Design review of the part built by this model. Coordinates are the model's own, in mm. Face numbers are marked on the shaded views. A direction names the side the tool comes from. Coordinates: 2 decimals unless noted, no trailing zeros. Write each loop counter-clockwise with the first axis right and the second up, starting at its lowest first coordinate (ties: lowest second). Pieces come first, ordered by that corner, then holes. Notation, with made-up numbers: (9, 37.5) - (64, 37.5) arc R32 ccw to (64, 71.5) - close; hole circle Ø8 at (20, 82). An arc over 180 degrees is marked (long way). Use a Markdown table: item, result.
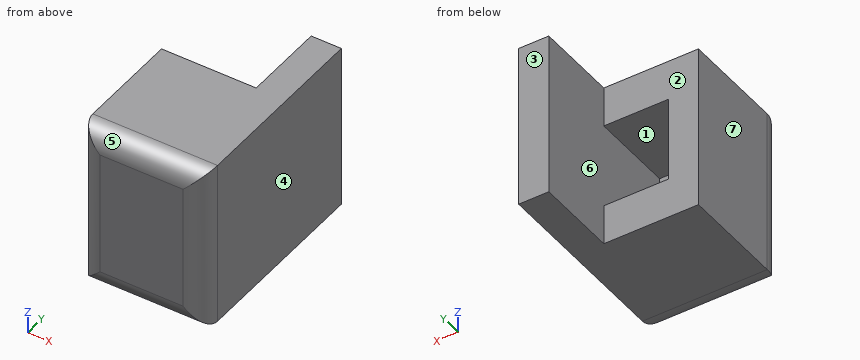
Autodesk Inventor part; units mm, degrees
ref_plane "YZ Plane" through (0, 0, 0) normal (1, 0, 0) x (0, 1, 0)
ref_plane "XZ Plane" through (0, 0, 0) normal (0, 1, 0) x (-1, 0, 0)
ref_plane "XY Plane" through (0, 0, 0) normal (0, 0, 1) x (1, 0, 0)
sketch "Sketch1" plane through (0, 0, 0) normal (0, 1, 0) x (-1, 0, 0)
  line L0 (15, 20) -> (-15, 20)
  line L1 (-15, 20) -> (-15, -20)
  line L2 (-15, -20) -> (15, -20)
  line L3 (15, -20) -> (15, 20)
  line L4 (15, 20) -> (-15, -20) construction
  line L5 (-15, 20) -> (15, -20) construction
  point P0 (0, 0)
  dimension "d0" = 30
  dimension "d1" = 40
extrude "Extrusion1" add sketch "Sketch1" along normal blind 50
sketch "Sketch2" plane through (0, 50, 0) normal (0, 1, 0) x (1, 0, 0)
  line L0 (-7.75, -25.4) -> (7.75, -25.4)
  line L1 (7.75, -25.4) -> (7.75, 25.4)
  line L2 (7.75, 25.4) -> (-7.75, 25.4)
  line L3 (-7.75, 25.4) -> (-7.75, -25.4)
  line L4 (-7.75, -25.4) -> (7.75, 25.4) construction
  line L5 (7.75, -25.4) -> (-7.75, 25.4) construction
  point P0 (0, 0)
  dimension "d4" = 15.5
extrude "Extrusion2" cut sketch "Sketch2" against normal blind 20
sketch "Sketch3" plane through (0, 30, 0) normal (0, 1, 0) x (1, 0, 0)
  line L0 (-7.75, -10.25) -> (7.75, -10.25)
  line L1 (7.75, -10.25) -> (7.75, 10.25)
  line L2 (7.75, 10.25) -> (-7.75, 10.25)
  line L3 (-7.75, 10.25) -> (-7.75, -10.25)
  line L4 (-7.75, -10.25) -> (7.75, 10.25) construction
  line L5 (7.75, -10.25) -> (-7.75, 10.25) construction
  point P0 (0, 0)
  dimension "d7" = 15.5
  dimension "d8" = 20.5
extrude "Extrusion3" cut sketch "Sketch3" against normal blind 20.3
fillet "Fillet1" radius 5 4 edges at (15, 0, 0) (-15, 0, 0) (0, 0, 20) (0, 0, -20)
sketch "Sketch4" plane through (0, 50, 0) normal (0, 1, 0) x (1, 0, 0)
  line L0 (-7.75, -20) -> (-7.75, 20)
  line L1 (-7.75, 20) -> (-15, 20)
  line L2 (-15, 20) -> (-15, -20)
  line L3 (-15, -20) -> (-7.75, -20)
  point P0 (0, 0)
extrude "Extrusion4" cut sketch "Sketch4" against normal blind 20
properties part number "SEGURO DE GUIA DE TAPA PRINCIPAL"
(1) Machinability: for the marked faces 1, 2 and 3, which of the approach directions +Z, -Z, +X, -X, +Y, -Y give a long, thin tool a straight path to every point of the face, cutting with its end or side? Answer none if there is none.
Determined:
| item | result |
|---|---|
| face 1 | +Y |
| face 2 | +Z, -Z, -X, +Y |
| face 3 | +Z, -Z, +X, -X, +Y |
(2) Take a section at A-A on y = 29. Write out the cut boundary in (x, z), and give its area (3 significant figures).
Determined:
| item | result |
|---|---|
| outline | (-15, -20) - (15, -20) - (15, 20) - (-15, 20) - close; hole (-7.75, -10.25) - (7.75, -10.25) - (7.75, 10.25) - (-7.75, 10.25) - close |
| area | 882 mm2 |
(3) For L1, parallel to X at y = 21, z = 5.5; L2, parallel to X at y = 36, z = 6.5; L3, parallel to Y at x = 3.5, z = 6.5, list the stretches that pass through material, from the lowest coordinate up. Write a range as from..to.
Determined:
| item | result |
|---|---|
| L1 | -15..-7.75, 7.75..15 |
| L2 | 7.75..15 |
| L3 | 0..9.7 |
(4) Take a section at B-B on z = -11. Write out the cut boundary in (x, y), and give its area (3 significant figures).
Determined:
| item | result |
|---|---|
| outline | (-15, 5) arc R5 ccw to (-10, 0) - (10, 0) arc R5 ccw to (15, 5) - (15, 50) - (7.75, 50) - (7.75, 30) - (-15, 30) - close |
| area | 1,030 mm2 |
(5) Draft analysis for pull direction X (two halves, no side actions). For the marked faces 4, 5, 6 and 7, state which applies: +X half, -X half, draft (parallel to the pull), parting line (faces both ways), or undercut.
Determined:
| item | result |
|---|---|
| face 4 | +X half |
| face 5 | draft |
| face 6 | undercut |
| face 7 | -X half |
(6) For pin 1 (12.5 mm diameter, centred on x = -3.5, z = 2.5, fed in from +Y); pin 2 (4 mm diameter, centred on x = 2, z = -0.5, fed in from +Y), all flat-tipped, find the tip position at first contact; note any pin that passes through.
Determined:
| item | result |
|---|---|
| pin 1 | y = 30 |
| pin 2 | y = 9.7 |
(7) Take a section at C-C on x = -2.5. Write out the cut boundary in (y, z).
Determined:
| item | result |
|---|---|
| outline | (0, -15) arc R5 ccw to (5, -20) - (30, -20) - (30, -10.25) - (9.7, -10.25) - (9.7, 10.25) - (30, 10.25) - (30, 20) - (5, 20) arc R5 ccw to (0, 15) - close |
(8) Take a section at D-D on z = 9. Write out the cut boundary in (x, y).
Determined:
| item | result |
|---|---|
| outline | (-15, 5) arc R5 ccw to (-10, 0) - (10, 0) arc R5 ccw to (15, 5) - (15, 50) - (7.75, 50) - (7.75, 9.7) - (-7.75, 9.7) - (-7.75, 30) - (-15, 30) - close |
